Geometry: final body of the model. Coordinates: model frame, mm. Face numbers are marked on the shaded views. Give positions to 0.01 mm unless a question says otherwise; leave off trailing zeros. Use CSV: the item, a comma, the result in double quotes. Start each with the question number.
1) Material intervals for line 1 (Z direction, x = 12, y = 51); line 2 (X direction, y = 32, z = 52.5); line 3 (X direction, y = -10, z = 80.5), sorted ascending. Write a range as [from, to].
2) Draft query along Z for the marked faces 1 and 2. Return one class per face: pulls with the +Z half, pulls with the -Z half, needs draft (parallel to the pull), parting line crosses it, or undercut.
3) Contact query for flat-ended pins moving along their axis: P1, Ø2, axis at x = -26.5, y = 71.5, coming from the -Z side; P2, Ø5, axis at x = 46.5, y = 24, coming from the +Z side; P3, Ø3, axis at x = -7.5, z = -35, coming from the +Y side. Output: stop coordinate, or through.
```python
from build123d import *

# Parameters (mm, degrees)
F2_T = -2.54


with BuildPart() as f1:
    # F0 (on Top) → F1 (revolve)
    with BuildSketch(Plane.XY):
        Polygon((-0.917275699, 61.8508926201), (-54.0230821053, 30.1310622525), (-53.1058064063, -31.7198303677), (0.917275699, -61.8508926201), (54.0230821053, -30.1310622525), (53.1058064063, 31.7198303677), align=None)
    revolve(axis=Axis((26.0942653536, 46.7853614939, 0), (0.8733445845, -0.4871029015, 0)))

    # F2 (hollow: no face is removed)
    offset(amount=F2_T, mode=Mode.SUBTRACT)


solid = f1.part
```
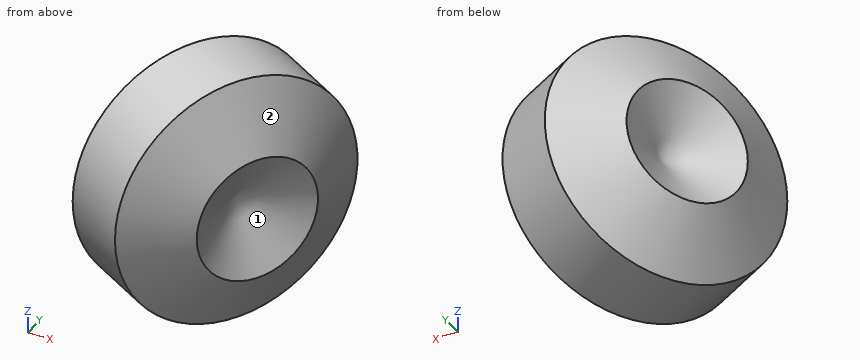
Answers follow:
1,line 1,"z = [-107.09, -104.55], [104.55, 107.09]"
1,line 2,"x = [-42.18, -39.4], [84.53, 87.6]"
1,line 3,"x = [-17.24, -9.21], [36.49, 40.46]"
2,face 1,"undercut"
2,face 2,"parting line crosses it"
3,P1,"stops at z = -61.9"
3,P2,"stops at z = 106.88"
3,P3,"stops at y = 114.13"
